Geometry: final body of the model. Coordinates: model frame, mm. Face numbers are marked on the shaded views. Coordinates: 2 decimals unless noted, no trailing zeros. Order: outer loops, then holes, each group sorted by start corner. A loop starts at its lowest first (then second) coordinate and runs counter-clockwise, first axis right, second up. Notation, with made-up numbers: M -32,0 L 11,0 A22 cw 11,30 Z; hole C 19,-13.75 d1. An arc over 180 degrees is marked long. One line per question, with ' | ' between items.
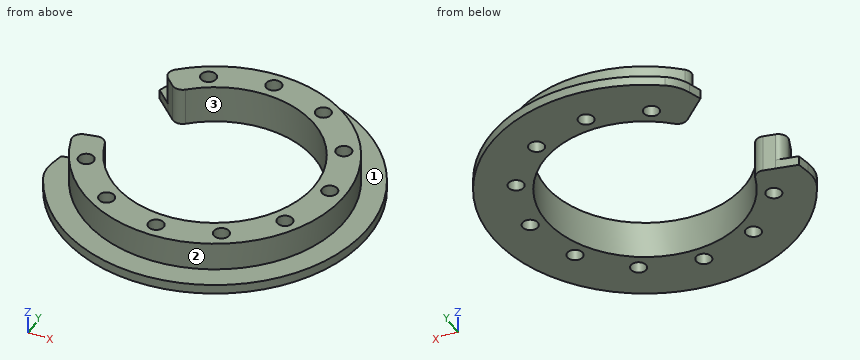
Autodesk Inventor part; units mm, degrees
ref_plane "YZ Plane" through (0, 0, 0) normal (1, 0, 0) x (0, 1, 0)
ref_plane "XZ Plane" through (0, 0, 0) normal (0, 1, 0) x (-1, 0, 0)
ref_plane "XY Plane" through (0, 0, 0) normal (0, 0, 1) x (1, 0, 0)
sketch "Sketch1" plane through (0, 0, 0) normal (0, 0, 1) x (1, 0, 0)
  circle A0 centre (0, 38.1) radius 2.54
  circle A1 centre (-19.05, 32.9956) radius 2.54
  circle A2 centre (-32.9956, 19.05) radius 2.54
  circle A3 centre (-38.1, 0) radius 2.54
  arc A4 (-34.7393, -15.6458) -> (-25.6134, 28.2057) centre (0, 0) ccw
  line L0 (0, 0) -> (-22.4665, 0)
  arc A5 (-42.1565, -9.3459) -> (-31.8356, 29.172) centre (0, 0) ccw
  arc A6 (-32.2373, -7.1468) -> (-24.3449, 22.308) centre (0, 0) ccw
  line L1 (-31.8356, 29.172) -> (-24.3449, 22.308)
  line L2 (-42.1565, -9.3459) -> (-32.2373, -7.1468)
  circle A7 centre (-32.9956, -19.05) radius 2.54
  circle A8 centre (-19.05, -32.9956) radius 2.54
  circle A9 centre (0, -38.1) radius 2.54
  circle A10 centre (19.05, -32.9956) radius 2.54
  circle A11 centre (32.9956, -19.05) radius 2.54
  circle A12 centre (38.1, 0) radius 2.54
  circle A13 centre (32.9956, 19.05) radius 2.54
  circle A14 centre (19.05, 32.9956) radius 2.54
  dimension "d0" = 38.1
  dimension "d3" = 360
  dimension "d5" = 5.08
  dimension "d6" = 5.08
  dimension "d7" = 5.08
  dimension "d8" = 55
  dimension "d9" = 42.5
extrude "Extrusion1" add sketch "Sketch1" along normal blind 12.7 contours L2 A6 L1 A5
fillet "Fillet2" radius 3.175 4 edges at (-31.8356, 29.172, 6.35) (-24.3449, 22.308, 6.35) (-32.2373, -7.1468, 6.35) (-42.1565, -9.3459, 6.35)
sketch "Sketch2" plane through (0, 0, 0) normal (0, 0, -1) x (-1, 0, 0)
  arc A0 (29.42, 31.6066) -> (41.2817, -12.6621) centre (0, 0) ccw
  arc A1 (37.4537, 34.32) -> (49.5958, -10.9951) centre (0, 0) ccw
  line L0 (37.4537, 34.32) -> (29.4017, 26.9417)
  line L1 (29.4017, 26.9417) -> (26.5829, 24.3587)
  arc A2 (29.4017, 26.9417) -> (29.42, 31.6066) centre (27.2567, 29.2826) ccw
  line L2 (35.2008, -7.8038) -> (38.9335, -8.6314)
  arc A3 (41.2817, -12.6621) -> (38.9335, -8.6314) centre (38.2463, -11.7311) ccw
  line L3 (49.5958, -10.9951) -> (38.9335, -8.6314)
  dimension "d20" = 50.8
extrude "Extrusion2" add sketch "Sketch2" against normal blind 3.175
chamfer "Chamfer3" distance 7.62 distance2 3.81 1 edges at (-37.4537, 34.32, 1.5875) measured on face at (-32.5487, -39.0029, 2.1167)
chamfer "Chamfer4" distance 3.81 distance2 7.62 1 edges at (-49.5958, -10.9951, 1.5875) measured on face at (-36.4451, -8.0797, 5.2917)
fillet "Fillet3" radius 12.7 2 edges at (-47.3933, -18.2899, 1.5875) (-31.8988, 39.5361, 1.5875)
equation "\"d7\" = d6"
properties part number "RotateLimitPlate"
1. Material intervals for line 1 (Y direction, x = 0, z = 3.5); line 2 (Y direction, x = 19.05, z = 4.25); line 3 (X direction, y = 0, z = 9.75), sorted ascending. Write a range as [from, to].
Response values:
line 1: y = [-43.18, -40.64], [-35.56, -33.02], [33.02, 35.56], [40.64, 43.18] | line 2: y = [-38.75, -35.54], [-30.46, -26.97], [26.97, 30.46], [35.54, 38.75] | line 3: x = [33.02, 35.56], [40.64, 43.18]
2. Draft query along X for the marked faces 1, 2 and 3. Return one class per face: pulls with the +X half, pulls with the -X half, needs draft (parallel to the pull), parting line crosses it, or undercut.
Response values:
face 1: needs draft | face 2: parting line crosses it | face 3: undercut
3. Pin query (flat end, axial travel): P1, Ø1, axis at y = -27, z = 4, coming from the +X side; P2, Ø2, axis at x = -9, z = 6, coming from the -Y side; P3, Ø4, axis at y = -34, z = 4, coming from the -X side. Return the tip coordinate at first contact, or that it passes through.
Response values:
P1: stops at x = 34.09 | P2: stops at y = -42.43 | P3: stops at x = -39.31
4. Section C-C, the plane x = 10.5. Output: boundary loops of the cut face in (y, z) (3 decimals).
Response values:
outline: M -49.703,0 L -31.306,0 L -31.306,12.7 L -41.884,12.7 L -41.884,3.175 L -49.703,3.175 Z; M 31.306,0 L 49.703,0 L 49.703,3.175 L 41.884,3.175 L 41.884,12.7 L 31.306,12.7 Z
5. Section A-A, the plane y = 0. Output: boundary loops of the cut face in (x, z) (3 decimals).
Response values:
outline: M 33.02,0 L 35.56,0 L 35.56,12.7 L 33.02,12.7 Z; M 40.64,0 L 50.8,0 L 50.8,3.175 L 43.18,3.175 L 43.18,12.7 L 40.64,12.7 Z
6. Section B-B, the plane x = 0. Output: boundary loops of the cut face in (y, z) (3 decimals), and give its area (3 significant figures).
Response values:
outline: M -50.8,0 L -40.64,0 L -40.64,12.7 L -43.18,12.7 L -43.18,3.175 L -50.8,3.175 Z; M -35.56,0 L -33.02,0 L -33.02,12.7 L -35.56,12.7 Z; M 33.02,0 L 35.56,0 L 35.56,12.7 L 33.02,12.7 Z; M 40.64,0 L 50.8,0 L 50.8,3.175 L 43.18,3.175 L 43.18,12.7 L 40.64,12.7 Z | area: 177 mm^2
7. Section D-D, the plane z = 4.5. Give the number of separate pieces and of enclosed holes in the cut face, and give its area (3 significant figures).
Response values:
separate pieces: 1 | enclosed holes: 10 | area: 1,850 mm^2
